Input: part model. Units: mm. Frame: model coordinates. A direction names the side the tool comes from. Give positions to 0.01 mm unless a question says otherwise; leave off trailing zeros. Use a Markdown table: item, result. Add a question column.
1. Mould query, pull axis X, two halves, no side actions, for faces 1 (the flat face through (0, 5, -22.5)), 2 (the flat face through (-4, 5, 14)). Classes: released by +X, released by -X, zero draft, split by the parting line, or undercut.
2. Set-up query: faces 3 (the flat face through (1, 10, 1)), 4 (the flat face through (4, 5, 14)). Return all of +Z, -Z, +X, -X, +Y, -Y with unobstructed straight access to the full face (end or side cutting, diameter ignored); none if empty.
3. Pin query (flat end, axial travel): pin 1 (4 mm diameter, centred on x = -10, y = 2, fed in from +Z); pin 2 (2 mm diameter, centred on x = -23, y = 7.5, fed in from -Z); pin 3 (1.5 mm diameter, centred on x = -37, y = 7.5, fed in from +Z). Return the tip coordinate at first contact, or that it passes through.
4. Material intervals for probe 1 along X at (y, z) = (2.5, 6); probe 2 along X at (y, z) = (5, 8); probe 3 along Z at (x, y) = (-37.5, 8.5), sorted ascending.
```python
from build123d import *

# Parameters (mm, degrees)
BOSS_EXTRUDE1_DEPTH = 10
SKETCH5_W           = 8
SKETCH5_H           = 30
CUT_EXTRUDE4_DEPTH  = 10
FILLET12_R          = 4


with BuildPart() as part:
    # Sketch1 → Boss-Extrude1 (new body)
    with BuildSketch(Plane(origin=(0, 0, 0), x_dir=(1, 0, 0), z_dir=(0, 1, 0))):
        with BuildLine():
            Line((-21.794494718, 22.5), (21.794494718, 22.5))
            add(Edge.make_bspline(
                [(-21.794494718, 22.5), (-78.136825066, 8.856081987), (-39.068412533, -15.601755848), (0, -40.059593683), (39.068412533, -15.601755848), (78.136825066, 8.856081987), (21.794494718, 22.5)],
                knots=[2.021823139, 2.021823139, 2.021823139, 3.8155337, 3.8155337, 5.609244261, 5.609244261, 7.402954822, 7.402954822, 7.402954822], degree=2, weights=[1, 0.624070234, 1, 0.624070234, 1, 0.624070234, 1]))
        make_face()
    extrude(amount=BOSS_EXTRUDE1_DEPTH)

    # Sketch5 → Cut-Extrude4 (cut)
    with BuildSketch(Plane(origin=(0, 10, 0), x_dir=(1, 0, 0), z_dir=(0, 1, 0))):
        with Locations((0, -17.5)):
            Rectangle(SKETCH5_W, SKETCH5_H)
    extrude(amount=-CUT_EXTRUDE4_DEPTH, mode=Mode.SUBTRACT)

    # Fillet12
    fillet12_edges = [part.edges().sort_by_distance(p)[0] for p in [
        (47.117377831, 10, 8.365893651),
        (0, 0, -22.5),
        (-47.117377875, 0, 8.365893589),
        (-47.117377875, 10, 8.365893589),
        (0, 10, -22.5),
        (47.117377831, 0, 8.365893651),
    ]]
    fillet(fillet12_edges, radius=FILLET12_R)


solid = part.part
```
Result sheet:
| question | item | result |
|---|---|---|
| 1 | face 1 | zero draft |
| 1 | face 2 | undercut |
| 2 | face 3 | +Z, -Z, +X, -X, +Y |
| 2 | face 4 | +Z, +Y, -Y |
| 3 | pin 1 | stops at z = 24.59 |
| 3 | pin 2 | stops at z = -22.3 |
| 3 | pin 3 | stops at z = 16.98 |
| 4 | probe 1 | x = -48.21 to -4, 4 to 48.21 |
| 4 | probe 2 | x = -47.37 to -4, 4 to 47.37 |
| 4 | probe 3 | z = -15.52 to 15.52 |
